Model file for the job. Use its own axes, mm. A direction names the side the tool comes from. Round coordinates to 2 decimals unless told otherwise and drop trailing zeros. Loops run counter-clockwise (first coordinate to the right, second up) from the corner with the lowest first, then second, coordinate; pieces in that order, holes last. Notation, with made-up numbers: M 25,71.5 L 45,71.5 A18 ccw 45,94.5 Z; hole C -2.5,-36 d1. An arc over 180 degrees is marked long. Use a Markdown table: item, result. Add a question column.
Q1. Pin check, flat tips, straight feed: pin 1 (2 mm diameter, centred on x = -281.5, z = -9.5, fed in from -Y); pin 2 (1.5 mm diameter, centred on x = -188, z = 4.5, fed in from -Y); pin 3 (12 mm diameter, centred on x = -69, y = -82, fed in from -Z). Stop position of each tip, or through.
Q2. Mould opens along X. For faces 1 (the face through (-128.619, -80.145, 0.352)), 2 (the face through (-1.73, -34.06, -7.81)), 3 (the face through (-296.613, -92.983, -10.056)) say: +X half, -X half, draft (parallel to the pull), parting line (faces both ways), or undercut.
Q3. Cut at A-A (x = -26). Give the cut face in (y, z), plus the area to 3 significant figures.
Q4. Probe line 1 (Z direction, x = 0, y = -34); line 2 (Y direction, x = -179, z = -4); line 3 (Y direction, x = -215.5, z = -2) (3 decimals). List the from-to ranges inside material, lowest first. Write a range as from..to.
Q5. Tool access for faces 4 (the face through (-322.368, -93.4, -11.5)), 5 (the face through (-0.661, -34.06, 5.037)), 6 (the face through (5, 0, -2)), 7 (the face through (-296.613, -80.145, -11.23)), 8 (the face through (-128.619, -92.983, 1.526)): list every direction of +Z, -Z, +X, -X, +Y, -Y with a clear straight run to the whole face (end or side of a thin tool).
Q6. Cut at B-B (y = -18). Give the cut face in (x, z), plus the area to 3 significant figures.
from build123d import *

# Parameters (mm, degrees)
F0_R      = 8.001
F0_R_2    = 5.08
F1_DEPTH  = 69.088
F2_R      = 8.001
F2_R_2    = 5.08
F3_ANGLE  = 90
F4_R      = 8.001
F4_R_2    = 5.08
F5_DEPTH  = 222.25
F6_R      = 8.001
F6_R_2    = 5.08
F7_ANGLE  = 30
F8_R      = 8.001
F8_R_2    = 5.08
F9_DEPTH  = 12.954
F10_R     = 8.001
F10_R_2   = 5.08
F11_ANGLE = 30
F12_R     = 8.001
F12_R_2   = 5.08
F13_DEPTH = 50.8


with BuildPart() as f1:
    # F0 (on Front) → F1 (new body)
    with BuildSketch(Plane.XZ):
        Circle(F0_R)
        Circle(F0_R_2, mode=Mode.SUBTRACT)
    extrude(amount=F1_DEPTH)

    # F2 (on face) → F3 (revolve)
    with BuildSketch(Plane.XZ.offset(69.088)):
        Circle(F2_R)
        Circle(F2_R_2, mode=Mode.SUBTRACT)
    revolve(axis=Axis((-19.05, -69.088, 2.9448331334), (0, 0, -1)), revolution_arc=F3_ANGLE)

    # F4 (on face) → F5 (join)
    with BuildSketch(Plane(origin=(-19.05, 0, 0), x_dir=(0, -1, 0), z_dir=(-1, 0, 0))):
        with Locations((88.138, 0)):
            Circle(F4_R)
        with Locations((88.138, 0)):
            Circle(F4_R_2, mode=Mode.SUBTRACT)
    extrude(amount=F5_DEPTH)

    # F6 (on face) → F7 (revolve)
    with BuildSketch(Plane(origin=(-241.3, 0, 0), x_dir=(0, -1, 0), z_dir=(-1, 0, 0))):
        with Locations((88.138, 0)):
            Circle(F6_R)
        with Locations((88.138, 0)):
            Circle(F6_R_2, mode=Mode.SUBTRACT)
    revolve(axis=Axis((-241.3, -89.2251888638, -19.05), (0, -1, 0)), revolution_arc=F7_ANGLE)

    # F8 (on face) → F9 (join)
    with BuildSketch(Plane(origin=(-189.223891971, 0, -109.2484649666), x_dir=(0, -1, 0), z_dir=(-0.8660254038, 0, -0.5))):
        with Locations((88.138, 123.2022160579)):
            Circle(F8_R)
        with Locations((88.138, 123.2022160579)):
            Circle(F8_R_2, mode=Mode.SUBTRACT)
    extrude(amount=F9_DEPTH)

    # F10 (on face) → F11 (revolve)
    with BuildSketch(Plane(origin=(-200.4423850517, 0, -115.7254649666), x_dir=(0, -1, 0), z_dir=(-0.8660254038, 0, -0.5))):
        with Locations((88.138, 123.2022160579)):
            Circle(F10_R)
        with Locations((88.138, 123.2022160579)):
            Circle(F10_R_2, mode=Mode.SUBTRACT)
    revolve(axis=Axis((-271.5684930806, -88.2795984273, 7.4685678842), (0, 1, 0)), revolution_arc=F11_ANGLE)

    # F12 (on face) → F13 (join)
    with BuildSketch(Plane(origin=(-271.5684930806, 0, 0), x_dir=(0, -1, 0), z_dir=(-1, 0, 0))):
        with Locations((88.138, -11.5814321158)):
            Circle(F12_R)
        with Locations((88.138, -11.5814321158)):
            Circle(F12_R_2, mode=Mode.SUBTRACT)
    extrude(amount=F13_DEPTH)


solid = f1.part
Checked values:
| question | item | result |
|---|---|---|
| 1 | pin 1 | stops at y = -96.07 |
| 1 | pin 2 | stops at y = -95.21 |
| 1 | pin 3 | stops at z = -8 |
| 2 | face 1 | undercut |
| 2 | face 2 | parting line |
| 2 | face 3 | draft |
| 3 | outline | C -88.14,0 d16; hole C -88.14,0 d10.16 |
| 3 | area | 120 mm^2 |
| 4 | line 1 | z = -8..-5.08, 5.08..8 |
| 4 | line 2 | y = -95.07..-91.27, -85.01..-81.21 |
| 4 | line 3 | y = -95.885..-92.808, -83.468..-80.391 |
| 5 | face 4 | +Z, -Z, -X, +Y, -Y |
| 5 | face 5 | +Y |
| 5 | face 6 | +Z, -Z, +X, -X, +Y |
| 5 | face 7 | -X |
| 5 | face 8 | none |
| 6 | outline | C 0,0 d16; hole C 0,0 d10.16 |
| 6 | area | 120 mm^2 |
